Model file for the job. Use its own axes, mm. Round coordinates to 2 decimals unless told otherwise and drop trailing zeros. Loops run counter-clockwise (first coordinate to the right, second up) from the corner with the lowest first, then second, coordinate; pieces in that order, holes last. Notation, with made-up numbers: (-31, 11.25) -> (9, 11.25) arc R22 cw to (9, 44.25) -> close; hole circle Ø3 at (41, 85.25). An arc over 180 degrees is marked (long way). Use a Markdown table: item, result.
from build123d import *

# Parameters (mm, degrees)
BOSS_EXTRUDE1_DEPTH = 0.6
CUT_EXTRUDE1_DEPTH  = 16.632018424


with BuildPart() as part:
    # Sketch1 → Boss-Extrude1 (new body)
    with BuildSketch(Plane.XY):
        Polygon((0, 0), (0, 10), (12, 10), (12, 0), (10.5, 0), (10.5, 7), (1.5, 7), (1.5, 0), align=None)
    extrude(amount=BOSS_EXTRUDE1_DEPTH)

    # Sketch2 → Cut-Extrude1 (cut, through all)
    with BuildSketch(Plane.XY.offset(0.6)):
        Polygon((10.5, 10), (12, 8.5), (12, 10), align=None)
    extrude(amount=-CUT_EXTRUDE1_DEPTH, mode=Mode.SUBTRACT)


solid = part.part
Q1. Band-saw the part on B-B, the plane z = 0.25. Give the cut face in (x, y), plus the area to 3 significant figures.
Results list:
| item | result |
|---|---|
| outline | (0, 0) -> (1.5, 0) -> (1.5, 7) -> (10.5, 7) -> (10.5, 0) -> (12, 0) -> (12, 8.5) -> (10.5, 10) -> (0, 10) -> close |
| area | 55.9 mm² |
Q2. Band-saw the part on D-D, the plane y = 9.5. Give the cut face in (x, z), plus the area to 3 significant figures.
Results list:
| item | result |
|---|---|
| outline | (0, 0) -> (11, 0) -> (11, 0.6) -> (0, 0.6) -> close |
| area | 6.60 mm² |
Q3. Band-saw the part on C-C, the plane x = 8. Give the cut face in (y, z).
Results list:
| item | result |
|---|---|
| outline | (7, 0) -> (10, 0) -> (10, 0.6) -> (7, 0.6) -> close |
Q4. Band-saw the part on A-A, the plane y = 2.5. Give the cut face in (x, z).
Results list:
| item | result |
|---|---|
| outline | (0, 0) -> (1.5, 0) -> (1.5, 0.6) -> (0, 0.6) -> close; (10.5, 0) -> (12, 0) -> (12, 0.6) -> (10.5, 0.6) -> close |
Q5. Drill centre lines: L1, parallel to X at y = 4, z = 0.15; L2, parallel to Y at x = 5, z = 0.3; L3, parallel to X at y = 9, z = 0.2. Where is each one in solid material? Low to high. Write a range as from..to.
Results list:
| item | result |
|---|---|
| L1 | x = 0..1.5, 10.5..12 |
| L2 | y = 7..10 |
| L3 | x = 0..11.5 |
